from build123d import *

# Parameters (mm, degrees)
SKETCH1_W                  = 17.5
SKETCH1_H                  = 10
BASE_FLANGE1_DEPTH         = 2
F_4_CLEARANCE_HOLE1_D      = 3.2639
F_4_CLEARANCE_HOLE1_DEPTH  = 2
F_4_CLEARANCE_HOLE1_TIP    = 0.980574487
EDGE_FLANGE1_DEPTH         = 17.5
EDGE_FLANGE2_DEPTH         = 17.5
F_10_CLEARANCE_HOLE1_D     = 5.1054
F_10_CLEARANCE_HOLE1_DEPTH = 2
F_10_CLEARANCE_HOLE1_TIP   = 1.533816902


# Sheet-metal steps are written as plain solids
with BuildPart() as part:
    # Sketch1 → Base-Flange1 (new body)
    with BuildSketch(Plane(origin=(0, 0, 0), x_dir=(1, 0, 0), z_dir=(0, 1, 0))):
        with Locations((-8.75, 5)):
            Rectangle(SKETCH1_W, SKETCH1_H)
    extrude(amount=-BASE_FLANGE1_DEPTH)

    # #4 Clearance Hole1
    with Locations(Plane.XZ.offset(2)):
        with Locations((-4, -5), (-13.5, -5)):
            Hole(F_4_CLEARANCE_HOLE1_D / 2, depth=F_4_CLEARANCE_HOLE1_DEPTH)
            with Locations((0, 0, -(F_4_CLEARANCE_HOLE1_DEPTH + F_4_CLEARANCE_HOLE1_TIP / 2))):  # 118° drill point
                Cone(0, F_4_CLEARANCE_HOLE1_D / 2, F_4_CLEARANCE_HOLE1_TIP, mode=Mode.SUBTRACT)

    # Edge-Flange1 section (across the edge) → Edge-Flange1 (add)
    with BuildSketch(Plane(origin=(-17.5, -2, -10.7366), x_dir=(0, 0, 1), z_dir=(1, 0, 0))):
        with BuildLine():
            Line((-2, 0.7366), (-2, 19))
            Line((-2, 19), (0, 19))
            Line((0, 19), (0, 0.7366))
            ThreePointArc((0, 0.7366), (0.215745145, 0.215745145), (0.7366, 0))
            Line((0.7366, 0), (0.7366, -2))
            ThreePointArc((0.7366, -2), (-1.198468417, -1.198468417), (-2, 0.7366))
        make_face()
    extrude(amount=EDGE_FLANGE1_DEPTH)

    # Edge-Flange2 section (across the edge) → Edge-Flange2 (add)
    with BuildSketch(Plane(origin=(0, -21.7366, -12.7366), x_dir=(0, 1, 0), z_dir=(-1, 0, 0))):
        with BuildLine():
            Line((-2, 0.7366), (-2, 17.5))
            Line((-2, 17.5), (0, 17.5))
            Line((0, 17.5), (0, 0.7366))
            ThreePointArc((0, 0.7366), (0.215745145, 0.215745145), (0.7366, 0))
            Line((0.7366, 0), (0.7366, -2))
            ThreePointArc((0.7366, -2), (-1.198468417, -1.198468417), (-2, 0.7366))
        make_face()
    extrude(amount=EDGE_FLANGE2_DEPTH)

    # #10 Clearance Hole1
    with Locations(Plane.XZ.offset(23.7366)):
        with Locations((-8.75, -23.4732)):
            Hole(F_10_CLEARANCE_HOLE1_D / 2, depth=F_10_CLEARANCE_HOLE1_DEPTH)
            with Locations((0, 0, -(F_10_CLEARANCE_HOLE1_DEPTH + F_10_CLEARANCE_HOLE1_TIP / 2))):  # 118° drill point
                Cone(0, F_10_CLEARANCE_HOLE1_D / 2, F_10_CLEARANCE_HOLE1_TIP, mode=Mode.SUBTRACT)


solid = part.part
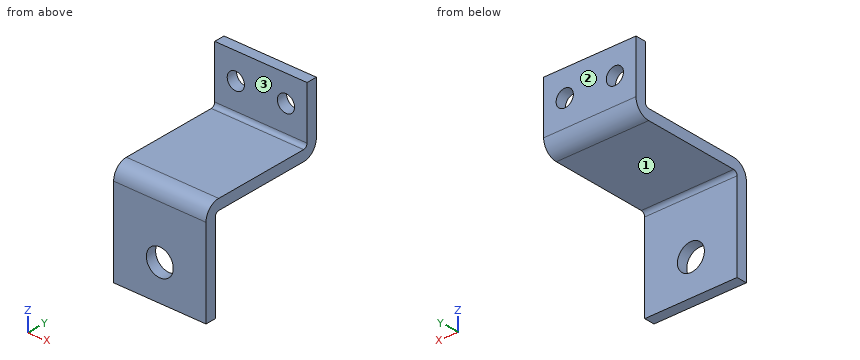
Verification items for the finished model (mm, model axes). Face numbers are marked on the shaded views. A direction names the side the tool comes from. Round coordinates to 2 decimals unless told otherwise and drop trailing zeros. Write each loop counter-clockwise with the first axis right and the second up, starting at its lowest first coordinate (ties: lowest second). Pieces come first, ordered by that corner, then holes.
(1) Section check A-A (x = -8.75). Enter the section's corners in (y, z), plus the area to 3 significant figures.
Returned:
outline: (-23.74, -30.24) - (-21.74, -30.24) - (-21.74, -26.03) - (-23.74, -26.03) - close; (-23.74, -20.92) - (-21.74, -20.92) - (-21.74, -13.47) arc R0.74 cw to (-21, -12.74) - (-2.74, -12.74) arc R2.74 ccw to (0, -10) - (0, 0) - (-2, 0) - (-2, -10) arc R0.74 cw to (-2.74, -10.74) - (-21, -10.74) arc R2.74 ccw to (-23.74, -13.47) - close
area: 90.8 mm2
(2) Section check D-D (z = -25.5). Enter the section's corners in (x, y), plus the area to 3 significant figures.
Returned:
outline: (-17.5, -23.74) - (-10.3, -23.74) - (-10.3, -21.74) - (-17.5, -21.74) - close; (-7.2, -23.74) - (0, -23.74) - (0, -21.74) - (-7.2, -21.74) - close
area: 28.8 mm2
(3) Access from +Z, -Z, +X, -X, +Y, -Y to the whole of each face (thin tool, end or side, straight path). Record for the marked faces 1, 2 and 3.
Returned:
face 1: -Z, +X, -X, +Y
face 2: +Z, -Z, +X, -X, +Y
face 3: +Z, +X, -X, -Y
(4) Material ranges on line 1 (X direction, y = -1, z = -5); line 2 (Y direction, x = -4.25, z = -16.5); line 3 (Z direction, x = -7, y = -18), recorded low to high.
Returned:
line 1: x = -17.5 to -15.13, -11.87 to -5.63, -2.37 to 0
line 2: y = -23.74 to -21.74
line 3: z = -12.74 to -10.74
(5) Section check C-C (x = -4). Enter the section's corners in (y, z).
Returned:
outline: (-23.74, -30.24) - (-21.74, -30.24) - (-21.74, -13.47) arc R0.74 cw to (-21, -12.74) - (-2.74, -12.74) arc R2.74 ccw to (0, -10) - (0, -6.63) - (-2, -6.63) - (-2, -10) arc R0.74 cw to (-2.74, -10.74) - (-21, -10.74) arc R2.74 ccw to (-23.74, -13.47) - close; (-2, -3.37) - (0, -3.37) - (0, 0) - (-2, 0) - close
(6) Depth check by flat-ended pin: pin 1 Ø6 at (x, z) = (-8.75, -23.47) entering from +Y; pin 2 Ø9 at (x, y) = (-7, -10.5) entering from +Z; pin 3 Ø3 at (x, z) = (-6.5, -6.5) entering from -Y; pin 4 Ø1 at (y, z) = (-19, -15) entering from -X. Enter the tip coordinate at first touch or a pass-through.
Returned:
pin 1: stops at y = -21.74
pin 2: stops at z = -10.74
pin 3: stops at y = -2
pin 4: passes through
(7) Section check B-B (z = -5). Enter the section's corners in (x, y), plus the area to 3 significant figures.
Returned:
outline: (-17.5, -2) - (-15.13, -2) - (-15.13, 0) - (-17.5, 0) - close; (-11.87, -2) - (-5.63, -2) - (-5.63, 0) - (-11.87, 0) - close; (-2.37, -2) - (0, -2) - (0, 0) - (-2.37, 0) - close
area: 21.9 mm2
